Geometry check sheet. Reference: the model listing, model coordinates, mm. A direction names the side the tool comes from. Give positions to 0.01 mm unless a question says otherwise; leave off trailing zeros. Order: outer loops, then holes, each group sorted by start corner. A loop starts at its lowest first (then second) coordinate and runs counter-clockwise, first axis right, second up.
from build123d import *

# Parameters (mm, degrees)
F0_W     = 70
F0_H     = 10.25
F0_H_2   = 17.5
F1_DEPTH = 10
F2_DEPTH = 3
F4_DEPTH = 25
F5_W     = 10
F5_H     = 94
F6_DEPTH = 90
F7_W     = 30
F7_H     = 5
F8_DEPTH = 20


with BuildPart() as f1:
    # F0 (on Front) → F1 (new body)
    with BuildSketch(Plane.XZ):
        with Locations((0, 13.875)):
            Rectangle(F0_W, F0_H)
        Rectangle(F0_W, F0_H_2)
        with Locations((0, -13.875)):
            Rectangle(F0_W, F0_H)
    extrude(amount=F1_DEPTH)

    # F0 (on Front) → F2 (join)
    with BuildSketch(Plane.XZ):
        Rectangle(F0_W, F0_H_2)
    extrude(amount=-F2_DEPTH)

    # F3 (on face) → F4 (cut)
    with BuildSketch(Plane.XZ.offset(10)):
        with BuildLine():
            ThreePointArc((-12.75, 0), (-13.40901, 1.59099), (-15, 2.25))
            ThreePointArc((-15, 2.25), (-17.235535, 0.254723), (-15.506171, -2.192325))
            Line((-15.506171, -2.192325), (-14.499388, -2.193601))
            ThreePointArc((-14.499388, -2.193601), (-13.240898, -1.402876), (-12.75, 0))
        make_face()
        with BuildLine():
            ThreePointArc((29.997148, -2.249998), (27.75, 0.001426), (30, 2.25))
            Line((30, 2.25), (-15, 2.25))
            ThreePointArc((-15, 2.25), (-13.40901, 1.59099), (-12.75, 0))
            ThreePointArc((-12.75, 0), (-13.240898, -1.402876), (-14.499388, -2.193601))
            Line((-14.499388, -2.193601), (29.997148, -2.249998))
        make_face()
        with BuildLine():
            ThreePointArc((29.997148, -2.249998), (31.589982, -1.591998), (32.25, 0))
            ThreePointArc((32.25, 0), (31.59099, 1.59099), (30, 2.25))
            ThreePointArc((30, 2.25), (27.75, 0.001426), (29.997148, -2.249998))
        make_face()
    extrude(amount=-F4_DEPTH, mode=Mode.SUBTRACT)

    # F5 (on face) → F6 (join)
    with BuildSketch(Plane.XZ.offset(10)):
        with Locations((-30, -28)):
            Rectangle(F5_W, F5_H)
    extrude(amount=F6_DEPTH)

    # F7 (on face) → F8 (join)
    with BuildSketch(Plane.YZ.offset(-25)):
        with Locations((-25, 16.5)):
            Rectangle(F7_W, F7_H)
        with Locations((-25, -16.5)):
            Rectangle(F7_W, F7_H)
    extrude(amount=F8_DEPTH)


solid = f1.part
Item 1: Scan lines: L1, parallel to Z at x = -22, y = -12; L2, parallel to X at y = -68.5, z = 13; L3, parallel to Y at x = -10.5, z = 2.5. Record each from-to range of solid material in increasing order.
Reported:
L1: z = -19 to -14, 14 to 19
L2: x = -35 to -25
L3: y = -10 to 3
Item 2: Gauge pin test, flat ends, axial feed: pin 1 (5.5 mm diameter, centred on x = -16, z = 16, fed in from -Y); pin 2 (1.5 mm diameter, centred on y = -27, z = -17, fed in from +X); pin 3 (19 mm diameter, centred on x = 3, z = 8, fed in from -Y); pin 4 (3.5 mm diameter, centred on x = 11.5, y = 1.5, fed in from +Z). Record the tip position at first contact, or that the pin passes through.
Reported:
pin 1: stops at y = -40
pin 2: stops at x = -5
pin 3: stops at y = -10
pin 4: stops at z = 19
Item 3: Sectioned sample at B-B (z = 10.5). Enter the section's corners in (x, y).
Reported:
outline: (-35, -100) - (-25, -100) - (-25, -10) - (35, -10) - (35, 0) - (-35, 0) - close
Item 4: Sectioned sample at D-D (y = -66.5). Enter the section's corners in (x, z), and give its area (3 significant figures).
Reported:
outline: (-35, -75) - (-25, -75) - (-25, 19) - (-35, 19) - close
area: 940 mm2
Item 5: Draft check along Z on faces 1 (the flat face through (0, 1, 8.75)), 2 (the flat face through (5, -10, 4)), 3 (the flat face through (-15, -25, -14)), 4 (the flat face through (-15, -40, 16)). Enter one of: released by +Z, released by -Z, zero draft, split by the parting line, or undercut.
Reported:
face 1: released by +Z
face 2: undercut
face 3: undercut
face 4: zero draft
Item 6: Sectioned sample at C-C (x = -22). Enter the section's corners in (y, z), and give its area (4 significant figures).
Reported:
outline: (-40, -19) - (0, -19) - (0, -8.75) - (3, -8.75) - (3, 8.75) - (0, 8.75) - (0, 19) - (-40, 19) - (-40, 14) - (-10, 14) - (-10, -14) - (-40, -14) - close
area: 732.5 mm2
Item 7: Sectioned sample at A-A (x = 8). Enter the section's corners in (y, z).
Reported:
outline: (-10, -19) - (0, -19) - (0, -8.75) - (3, -8.75) - (3, -2.22) - (-10, -2.22) - close; (-10, 2.25) - (3, 2.25) - (3, 8.75) - (0, 8.75) - (0, 19) - (-10, 19) - close
Item 8: Set-up check for faces 5 (the flat face through (8, -4, 2.25)), 6 (the flat face through (0, 1, -8.75)), 7 (the flat face through (-15, -40, -17)), 8 (the flat face through (0, 0, 14)): record each of +Z, -Z, +X, -X, +Y, -Y from which the full face is reachable in a straight line by a thin tool's end or side.
Reported:
face 5: +Y, -Y
face 6: -Z, +X, -X, +Y
face 7: +Z, -Z, +X, -Y
face 8: +Z, +X, -X, +Y
